The listing builds one solid part. Answer for the finished solid, in the listing's coordinates (mm). Face numbers are marked on the shaded views. A direction names the side the tool comes from. Coordinates: 2 decimals unless noted, no trailing zeros. Order: outer loops, then holes, each group sorted by start corner. A loop starts at its lowest first (then second) coordinate and runs counter-clockwise, first axis right, second up. Notation, with made-up numbers: (-25, 25.5) -> (-20, 25.5) arc R21 ccw to (-20, 55.5) -> close; hole circle Ø9 at (33, 85). An arc over 180 degrees is marked (long way). Write item = value, one per line.
from build123d import *

# Parameters (mm, degrees)
F1_DEPTH = 11
F2_R     = 1.25
F3_DEPTH = 22.001
F4_R     = 1.25
F5_DEPTH = 3.501
F6_SIZE  = 5.5
F7_W     = 5
F7_H     = 7
F8_DEPTH = 25


with BuildPart() as f1:
    # F0 (on Top) → F1 (new body, symmetric)
    with BuildSketch(Plane.XY):
        Polygon((11, 11), (8, 11), (8, -14), (-11, -14), (-11, -17.5), (11, -17.5), align=None)
    extrude(amount=F1_DEPTH, both=True)

    # F2 (on face) → F3 (cut, through all)
    with BuildSketch(Plane.YZ.offset(11)):
        with Locations((5.656854, -5.656854)):
            Circle(F2_R)
        with Locations((5.656854, 5.656854)):
            Circle(F2_R)
        with Locations((-5.656854, 5.656854)):
            Circle(F2_R)
        with Locations((-5.656854, -5.656854)):
            Circle(F2_R)
    extrude(amount=-F3_DEPTH, mode=Mode.SUBTRACT)

    # F4 (on face) → F5 (cut, through all)
    with BuildSketch(Plane(origin=(0, -14, 0), x_dir=(-1, 0, 0), z_dir=(0, 1, 0))):
        with Locations((5.656854, -5.656854)):
            Circle(F4_R)
        with Locations((5.656854, 5.656854)):
            Circle(F4_R)
        with Locations((-5.656854, 5.656854)):
            Circle(F4_R)
        with Locations((-5.656854, -5.656854)):
            Circle(F4_R)
    extrude(amount=-F5_DEPTH, mode=Mode.SUBTRACT)

    # F6
    f6_edges = [f1.edges().sort_by_distance(p)[0] for p in [
        (9.5, 11, 11),
        (9.5, 11, -11),
        (-11, -15.75, -11),
        (-11, -15.75, 11),
    ]]
    chamfer(f6_edges, length=F6_SIZE)

    # F7 (on face) → F8 (cut)
    with BuildSketch(Plane(origin=(8, 0, 0), x_dir=(0, -1, 0), z_dir=(-1, 0, 0))):
        with Locations((11.5, 0)):
            Rectangle(F7_W, F7_H)
    extrude(amount=-F8_DEPTH, mode=Mode.SUBTRACT)


solid = f1.part
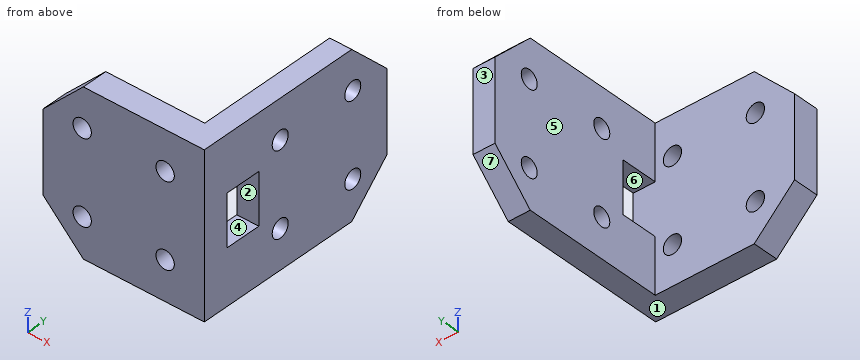
Q1. A tool of negligible diameter and unlimited length cuts with its end or side. For the marked faces 5, 6 and 7, from which of +Z, -Z, +X, -X, +Y, -Y can it reach the whole face along a straight path? Write none if from no direction.
The answers:
face_5 = +Z, -Z, -X, +Y
face_6 = +X, -X
face_7 = -Z, +X, -X, +Y
Q2. Each of these flat-tipped pins is pushed along its axis until it touches: pin 1 Ø4 at (y, z) = (-6.5, 1) entering from -X; pin 2 Ø4 at (x, z) = (5.66, -5.66) entering from +Y; pin 3 Ø10 at (x, y) = (-8.5, -14) entering from +Z; pin 4 Ø1.5 at (y, z) = (-5.66, -5.66) entering from -X. Where does it stop, or does it pass through?
The answers:
pin_1 = 8
pin_2 = -14
pin_3 = 11
pin_4 = through
Q3. Section B-B, the plane x = 6.25 is taken. Give the vertices of the cut face in (y, z), plus the area to 3 significant figures.
The answers:
outline = (-17.5, -11) -> (-14, -11) -> (-14, -6.76) -> (-17.5, -6.76) -> close; (-17.5, -4.56) -> (-14, -4.56) -> (-14, 4.56) -> (-17.5, 4.56) -> close; (-17.5, 6.76) -> (-14, 6.76) -> (-14, 11) -> (-17.5, 11) -> close
area = 61.6 mm2
Q4. Section C-C, the plane y = -4.75 is taken. Give the vertices of the cut face in (x, z), plus the area to 3 significant figures.
The answers:
outline = (8, -11) -> (11, -11) -> (11, -6.52) -> (8, -6.52) -> close; (8, -4.8) -> (11, -4.8) -> (11, 4.8) -> (8, 4.8) -> close; (8, 6.52) -> (11, 6.52) -> (11, 11) -> (8, 11) -> close
area = 55.7 mm2
Q5. Section D-D, the plane z = 6 is taken. Give the vertices of the cut face in (x, y), plus the area to 3 significant figures.
The answers:
outline = (-10.5, -17.5) -> (-6.86, -17.5) -> (-6.86, -14) -> (-10.5, -14) -> close; (-4.45, -17.5) -> (4.45, -17.5) -> (4.45, -14) -> (-4.45, -14) -> close; (6.86, -17.5) -> (11, -17.5) -> (11, -6.86) -> (8, -6.86) -> (8, -14) -> (6.86, -14) -> close; (8, -4.45) -> (11, -4.45) -> (11, 4.45) -> (8, 4.45) -> close; (8, 6.86) -> (11, 6.86) -> (11, 10.5) -> (8, 10.5) -> close
area = 117 mm2
Q6. Section A-A, the plane z = -0.75 is taken. Give the vertices of the cut face in (x, y), plus the area to 3 significant figures.
The answers:
outline = (-11, -17.5) -> (11, -17.5) -> (11, -14) -> (-11, -14) -> close; (8, -9) -> (11, -9) -> (11, 11) -> (8, 11) -> close
area = 137 mm2
Q7. Find the intervals of material crossed by line 1 along Z through (x, y) = (5.75, -15.75); line 2 along Y through (x, z) = (-1, 8); line 3 along X through (y, z) = (-8.5, 9.25), in increasing order.
The answers:
line_1 = -11 to -6.9, -4.41 to 4.41, 6.9 to 11
line_2 = -17.5 to -14
line_3 = 8 to 11
Q8. The mould has two halves that part along Y. Classify the marked faces 1, 2, 3 and 4: released by +Y, released by -Y, zero draft, split by the parting line, or undercut.
The answers:
face_1 = zero draft
face_2 = undercut
face_3 = released by +Y
face_4 = undercut
